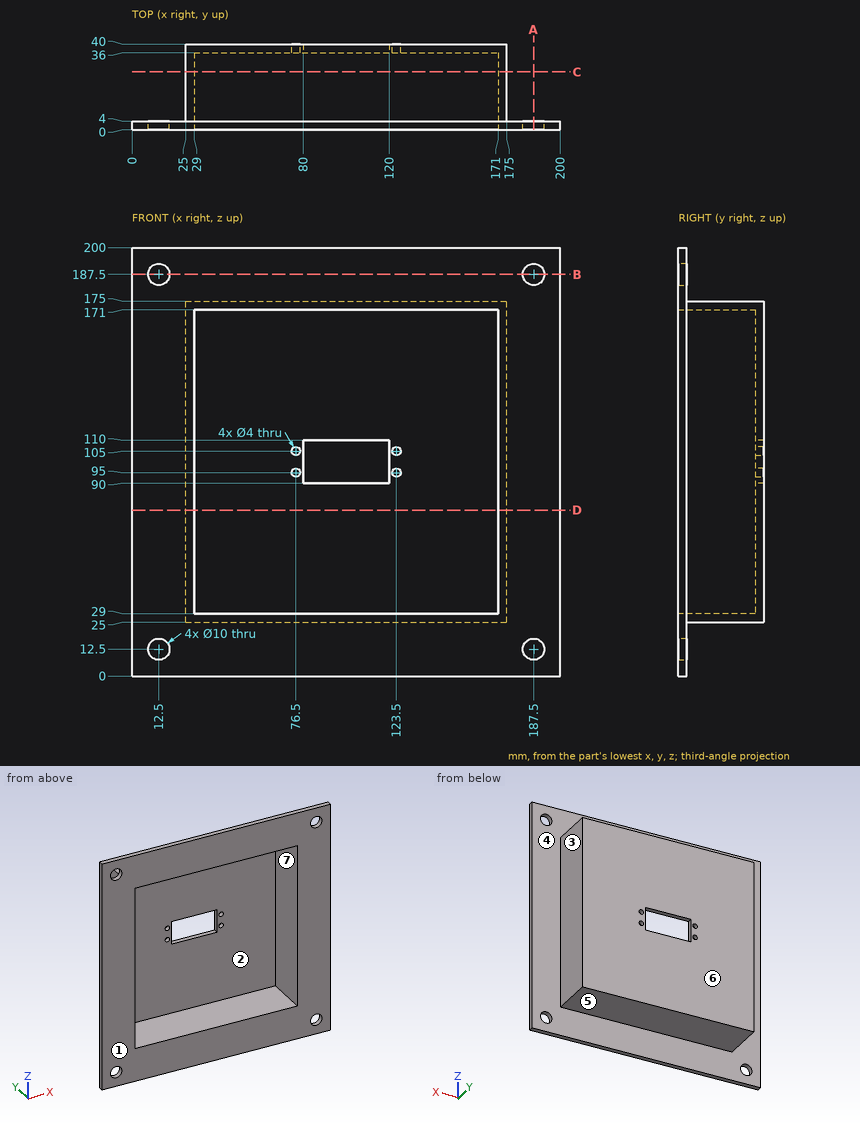
Study the drawing (mm; zero at the part's minimum x, y, z) and answer. A direction names the side the tool comes from. Round coordinates to 2 decimals unless told otherwise and drop trailing zeros. Write each loop counter-clockwise with the first axis right and the second up, starting at its lowest first coordinate (ties: lowest second). Pieces come first, ordered by that corner, then holes. Notation, with made-up numbers: (86, 51) - (140, 51) arc R34 cw to (140, 89) - close; hole circle Ø3 at (32.25, 14). An arc over 180 degrees is marked (long way). Return JSON: item names as keys, results as strings. Group by question number.
Q1. The part is cut by section B-B on z = 187.5. Write down the section's boundary in (x, y).
Q2. The part is cut by section D-D on z = 77.5. Write down the section's boundary in (x, y).
Q3. The mould has two halves that part along Z. Classify the marked faces 5, 6 and 7: released by +Z, released by -Z, zero draft, split by the parting line, or undercut.
Q4. Each of these flat-tipped pins is pushed along its axis until it touches: pin 1 Ø18 at (y, z) = (21.5, 65.5) entering from +X; pin 2 Ø18 at (y, z) = (21, 74) entering from -X; pin 3 Ø11 at (x, y) = (134.5, 17) entering from +Z; pin 4 Ø8 at (y, z) = (5, 118) entering from +X. Where does it stop, or does it pass through?
Q5. Find the intervals of material crossed by L1, parallel to X at y = 38.75, z = 95; L2, parallel to X at y = 2, z = 12, in increasing order.
Q6. The part is cut by section C-C on y = 27. Write down the section's boundary in (x, z).
Q7. For the marked faces 1, 2, 3 and 4, determine the directions among +Z, -Z, +X, -X, +Y, -Y from which every point of the face is accessible in a straight line to the end or side of a thin tool.
Q8. The part is cut by section A-A on x = 187.5. Write down the section's boundary in (y, z), then the cut area to 3 significant figures.
Solved:
{
 "1": {"outline": "(0, 0) - (7.5, 0) - (7.5, 4) - (0, 4) - close; (17.5, 0) - (182.5, 0) - (182.5, 4) - (17.5, 4) - close; (192.5, 0) - (200, 0) - (200, 4) - (192.5, 4) - close"},
 "2": {"outline": "(0, 0) - (29, 0) - (29, 36) - (171, 36) - (171, 0) - (200, 0) - (200, 4) - (175, 4) - (175, 40) - (25, 40) - (25, 4) - (0, 4) - close"},
 "3": {"face 5": "released by -Z", "face 6": "zero draft", "face 7": "undercut"},
 "4": {"pin 1": "x = 175", "pin 2": "x = 25", "pin 3": "z = 175", "pin 4": "x = 200"},
 "5": {"L1": "25 to 74.5, 78.5 to 80, 120 to 121.5, 125.5 to 175", "L2": "0 to 7.53, 17.47 to 182.53, 192.47 to 200"},
 "6": {"outline": "(25, 25) - (175, 25) - (175, 175) - (25, 175) - close; hole (29, 29) - (171, 29) - (171, 171) - (29, 171) - close"},
 "7": {"face 1": "+Z, -Z, +X, -X, -Y", "face 2": "-Y", "face 3": "+Z, -Z, +X, +Y", "face 4": "+Y"},
 "8": {"outline": "(0, 0) - (4, 0) - (4, 7.5) - (0, 7.5) - close; (0, 17.5) - (4, 17.5) - (4, 182.5) - (0, 182.5) - close; (0, 192.5) - (4, 192.5) - (4, 200) - (0, 200) - close", "area": "720 mm²"}
}
